Here's how the part is built. I have some questions about the finished solid (model axes, mm). Face numbers are marked on the shaded views. Coordinates: 2 decimals unless noted, no trailing zeros. Write each loop counter-clockwise with the first axis right and the second up, starting at its lowest first coordinate (ties: lowest second). Pieces come first, ordered by that corner, then holes. Notation, with made-up numbers: (52.5, -20.5) - (72.5, -20.5) arc R18 cw to (72.5, 13.5) - close; hole circle Ø7 at (-23.75, -23). An arc over 180 degrees is marked (long way). Answer in a Markdown table with one row per item. Add a question column.
Item 1: Imagine slicing it at C-C (z = 0.75). State how many separate pieces and enclosed holes the cut face has, plus the area to 3 significant figures.
Item 2: Imagine slicing it at D-D (x = -39). Please give me the cut outline in (y, z) (3 decimals).
Item 3: If I drill on probe 1 along Y at (x, z) = (-19.05, 1.35); probe 2 along X at (y, z) = (25, 0.65); probe 3 along X at (y, z) = (-17, 1.45), over which ranges is the centre line in solid material (lowest first)? Write a range as from..to.
Item 4: I'm going to push flat-ended pins straight in: pin 1 (3.5 mm diameter, centred on x = -19.05, y = 10.65, fed in from +Z); pin 2 (1 mm diameter, centred on y = -54, z = 1, fed in from -X). Where does each tip first touch, or does it pass through?
Item 5: Imagine slicing it at B-B (y = 9.5). Please give me the cut outline in (x, z) (3 decimals).
Item 6: We'd pull the mould along Z, two halves only. Please class the marked faces 1 and 2: +Z half, -Z half, draft (parallel to the pull), parting line (faces both ways), or undercut.
Item 7: Imagine slicing it at A-A (x = -19.05). Please give me the cut outline in (y, z) (3 decimals).
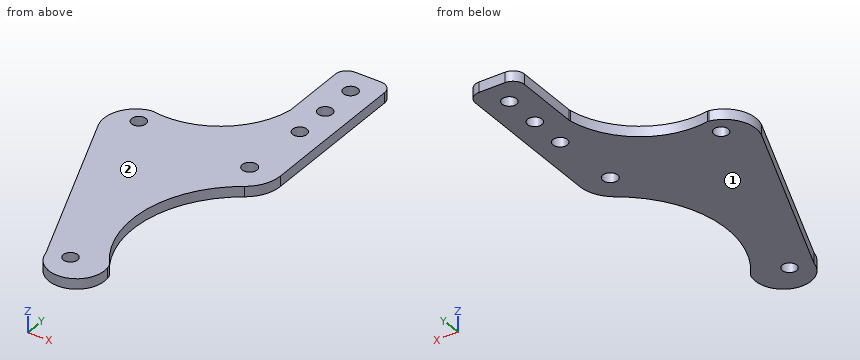
from build123d import *

# Parameters (mm, degrees)
SKETCH1_R           = 2.2225
BOSS_EXTRUDE1_DEPTH = 3.175
SKETCH2_R           = 2.286
CUT_EXTRUDE1_DEPTH  = 111.684893933


with BuildPart() as part:
    # Sketch1 → Boss-Extrude1 (new body)
    with BuildSketch(Plane.XY):
        with BuildLine():
            Line((-26.682968963, 26.357722587), (-26.682968963, 6.351785872))
            ThreePointArc((-26.682968963, 6.351785872), (-26.693527307, 6.120431356), (-26.725114563, 5.891000243))
            ThreePointArc((-26.725114563, 5.891000243), (-36.932915208, -9.945248539), (-55.328203965, -14.019474973))
            ThreePointArc((-55.328203965, -14.019474973), (-55.554473877, -14.001365453), (-55.780223055, -14.025100158))
            ThreePointArc((-55.780223055, -14.025100158), (-62.402560981, -18.816713415), (-63.103372405, -26.960654757))
            Line((-63.103372405, -26.960654757), (-40.595944625, -83.455943866))
            ThreePointArc((-40.595944625, -83.455943866), (-30.641352377, -90.339421853), (-23.75787439, -80.384829605))
            ThreePointArc((-23.75787439, -80.384829605), (-23.88583974, -79.549342433), (-24.280867854, -78.802103023))
            ThreePointArc((-24.280867854, -78.802103023), (-30.912062559, -52.492603109), (-16.357010265, -29.594721511))
            ThreePointArc((-16.357010265, -29.594721511), (-12.809669567, -25.627558214), (-11.528139151, -20.46231955))
            Line((-11.528139151, -20.46231955), (-11.528139151, 26.357722587))
            ThreePointArc((-11.528139151, 26.357722587), (-12.569667438, 28.872194301), (-15.084139151, 29.913722587))
            Line((-15.084139151, 29.913722587), (-23.126968963, 29.913722587))
            ThreePointArc((-23.126968963, 29.913722587), (-25.641440677, 28.872194301), (-26.682968963, 26.357722587))
        make_face()
        with Locations((-55.544078679, -19.824964902)):
            Circle(SKETCH1_R, mode=Mode.SUBTRACT)
        with Locations((-19.05, 22.084955235)):
            Circle(SKETCH1_R, mode=Mode.SUBTRACT)
        with Locations((-19.05, -0.775044765)):
            Circle(SKETCH1_R, mode=Mode.SUBTRACT)
        with Locations((-34.268702177, -81.651111456)):
            Circle(SKETCH1_R, mode=Mode.SUBTRACT)
        with Locations((-19.05, 10.654955235)):
            Circle(SKETCH1_R, mode=Mode.SUBTRACT)
    extrude(amount=BOSS_EXTRUDE1_DEPTH)

    # Sketch2 → Cut-Extrude1 (cut, through all)
    with BuildSketch(Plane.XY.offset(3.175)):
        with Locations((-20.267510202, -21.516890861)):
            Circle(SKETCH2_R)
    extrude(amount=-CUT_EXTRUDE1_DEPTH, mode=Mode.SUBTRACT)


solid = part.part
Here are the results:
| question | item | result |
|---|---|---|
| 1 | separate pieces | 1 |
| 1 | enclosed holes | 6 |
| 1 | area | 2,830 mm2 |
| 2 | outline | (-87.086, 0) - (-11.238, 0) - (-11.238, 3.175) - (-87.086, 3.175) - close |
| 3 | probe 1 | y = -31.63..-23.45, -19.58..-3, 1.45..8.43, 12.88..19.86, 24.31..29.91 |
| 3 | probe 2 | x = -26.68..-11.53 |
| 3 | probe 3 | x = -61.08..-11.53 |
| 4 | pin 1 | passes through |
| 4 | pin 2 | stops at x = -52.53 |
| 5 | outline | (-26.683, 0) - (-20.949, 0) - (-20.949, 3.175) - (-26.683, 3.175) - close; (-17.151, 0) - (-11.528, 0) - (-11.528, 3.175) - (-17.151, 3.175) - close |
| 6 | face 1 | -Z half |
| 6 | face 2 | +Z half |
| 7 | outline | (-31.63, 0) - (-23.452, 0) - (-23.452, 3.175) - (-31.63, 3.175) - close; (-19.582, 0) - (-2.998, 0) - (-2.998, 3.175) - (-19.582, 3.175) - close; (1.447, 0) - (8.432, 0) - (8.432, 3.175) - (1.447, 3.175) - close; (12.877, 0) - (19.862, 0) - (19.862, 3.175) - (12.877, 3.175) - close; (24.307, 0) - (29.914, 0) - (29.914, 3.175) - (24.307, 3.175) - close |
